Here's the drawing with two shaded views (mm, measured from the low corner). I have some questions. A direction names the side the tool comes from. Coordinates: 2 decimals unless noted, no trailing zeros. Write each loop counter-clockwise with the first axis right and the second up, starting at its lowest first coordinate (ties: lowest second). Pieces come first, ordered by that corner, then holes. Notation, with made-up numbers: M 37,34 L 62,34 A10 ccw 62,47 Z; hole C 6,-25.5 d3. An arc over 180 degrees is marked long. Use one line per item in the form item = value. Start each with the question number.
1. On a 3-axis mill with a long thin cutter (end or side, diameter ignored), from which of +Z, -Z, +X, -X, +Y, -Y can I reach the whole of each face in a straight line? I mean the marked faces 5, 6, 7 and 8. Say none if no direction works.
2. I'm going to push flat-ended pins straight in: pin 1 Ø0.8 at (x, y) = (11, 1.5) entering from -Z; pin 2 Ø1.4 at (x, z) = (11, 2.5) entering from -Y; pin 3 Ø0.7 at (y, z) = (1.5, 4) entering from -X; pin 4 Ø1 at (x, z) = (15, 4) entering from -Y. Where does each tip first touch, or does it pass through?
3. I want a section at C-C, the plane z = 2.85. List the corners of the cut face in (x, y) for me (3 decimals), plus the area to 4 significant figures.
4. I want a section at A-A, the plane y = 0.2. List the corners of the cut face in (x, z) for me, plus the area to 3 significant figures.
5. Please list where these lines run through material, in increasing order: line 1 along X through (y, z) = (1.5, 1.9); line 2 along X through (y, z) = (0.95, 2.5); line 3 along Z through (x, y) = (18.25, 0.9). Write a range as [from, to].
6. Thinking about a two-plate mould opening in X: for the marked faces 1, 2, 3 and 4, which applies, released by +X, released by -X, zero draft, split by the parting line, or undercut?
7. I want a section at D-D, the plane y = 1.8. List the corners of the cut face in (x, z) for me.
8. I want a section at B-B, the plane z = 4.45. List the corners of the cut face in (x, y) for me (3 decimals).
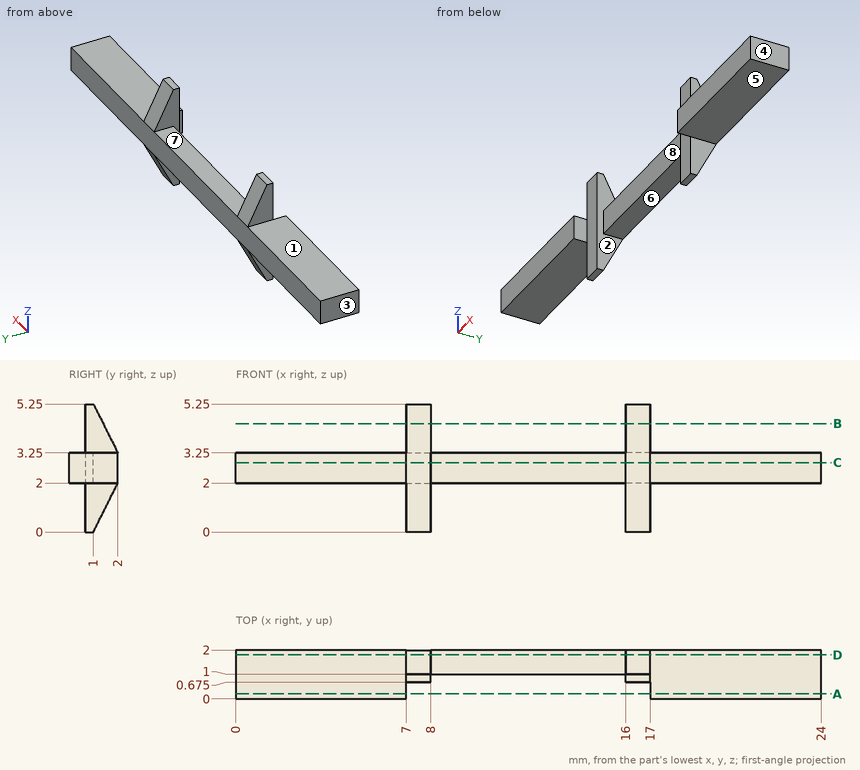
Answer list:
q1.face_5 = -Z, +X, +Y, -Y
q1.face_6 = -Z, +Y, -Y
q1.face_7 = +Z, +Y, -Y
q1.face_8 = +Z, -Z, -Y
q2.pin_1 = 2
q2.pin_2 = 1
q2.pin_3 = 7
q2.pin_4 = through
q3.outline = M 0,0 L 7,0 L 7,0.675 L 8,0.675 L 8,1 L 16,1 L 16,0.675 L 17,0.675 L 17,0 L 24,0 L 24,2 L 0,2 Z
q3.area = 38.65 mm²
q4.outline = M 0,2 L 7,2 L 7,3.25 L 0,3.25 Z; M 17,2 L 24,2 L 24,3.25 L 17,3.25 Z
q4.area = 17.5 mm²
q5.line_1 = [7, 8], [16, 17]
q5.line_2 = [0, 8], [16, 24]
q5.line_3 = [2, 3.25]
q6.face_1 = zero draft
q6.face_2 = undercut
q6.face_3 = released by -X
q6.face_4 = released by +X
q7.outline = M 0,2 L 7,2 L 7,1.6 L 8,1.6 L 8,2 L 16,2 L 16,1.6 L 17,1.6 L 17,2 L 24,2 L 24,3.25 L 17,3.25 L 17,3.65 L 16,3.65 L 16,3.25 L 8,3.25 L 8,3.65 L 7,3.65 L 7,3.25 L 0,3.25 Z
q8.outline = M 7,0.675 L 8,0.675 L 8,1.4 L 7,1.4 Z; M 16,0.675 L 17,0.675 L 17,1.4 L 16,1.4 Z
